```python
from build123d import *

# Parameters (mm, degrees)
F3_W     = 68.58
F3_H     = 68.58
F4_DEPTH = 48.1161598
F7_DEPTH = 203.2


with BuildPart() as f1:
    # F0 (on Front) → F1 (revolve)
    with BuildSketch(Plane.XZ):
        Polygon((228.6, 38.29685), (228.6, 63.5), (197.9639424, 63.5), (191.0935472, 51.6001), (81.237328, 51.6001), (79.8661598, 53.975), (48.1161598, 53.975), (48.1161598, 44.2595), (48.1161598, 38.29685), align=None)
        Polygon((48.1161598, 34.29), (48.1161598, 38.29685), (48.1161598, 44.2595), (0, 44.2595), (0, 34.29), align=None)
    revolve(axis=Axis((114.3, 0, 0), (1, 0, 0)))

    # F3 (on offset) → F4 (cut, through all)
    with BuildSketch(Plane(origin=(0, 0, 0), x_dir=(0, -1, 0), z_dir=(-1, 0, 0))):
        Rectangle(F3_W, F3_H)
    extrude(amount=-F4_DEPTH, mode=Mode.SUBTRACT)

    # F6 (on offset) → F7 (cut, symmetric)
    with BuildSketch(Plane(origin=(48.1161598, 0, 0), x_dir=(0, -1, 0), z_dir=(-1, 0, 0))):
        Polygon((-5.607271922, 5.607271922), (0, 0), (31.9966525594, 31.9966525594), (26.3893806374, 37.6039244814), align=None)
        Polygon((5.607271922, -5.607271922), (0, 0), (-5.607271922, 5.607271922), (-37.6039244814, -26.3893806374), (-26.3893806374, -37.6039244814), align=None)
        Polygon((31.9966525594, 31.9966525594), (0, 0), (5.607271922, -5.607271922), (37.6039244814, 26.3893806374), align=None)
    extrude(amount=F7_DEPTH, both=True, mode=Mode.SUBTRACT)


solid = f1.part
```
Work out the finished part from the listing and answer in its coordinate system (mm). A direction names the side the tool comes from. Give positions to 0.01 mm unless a question says otherwise; leave off trailing zeros. Loops run counter-clockwise (first coordinate to the right, second up) from the corner with the lowest first, then second, coordinate; pieces in that order, holes last. Notation, with made-up numbers: (65.25, 44.25) -> (76.25, 44.25) arc R13 cw to (76.25, 59.25) -> close; hole circle Ø1 at (-26.5, -8). An arc over 180 degrees is marked (long way). Put each result on its own line as item: value. Start each with the question number.
Item 1: Each of these flat-tipped pins is pushed along its axis until it touches: P1, Ø2, axis at y = -37, z = -1, coming from the +X side; P2, Ø3, axis at x = 96.5, y = 4.5, coming from the +Z side; P3, Ø0.7, axis at y = -33, z = 20.5, coming from the -X side. Where does it stop, or does it pass through?
Item 2: The part is cut by section A-A (z = 0). Give the vertices of the cut face in (x, y) (1 decimal), then the cut area to 3 significant figures.
Item 3: Which of the six approach directions +Z, -Z, +X, -X, +Y, -Y give full straight-line access (tool end or side, diameter ignored) to faces 4 (the face through (138.1, 34.814, -23.599)), 5 (the face through (24, -2, -34.29)), 6 (the face through (23.72, 44.24, 1.35)), 7 (the face through (24, 34.29, 2)), 8 (the face through (81.15, 50.52, -11.22))?
Item 4: The mould has two halves that part along Z. Classify faces 1 (the face through (139.62, 27.59, 26.56)), 2 (the face through (135.396, -15.499, 49.217)), 3 (the face through (0, -38, -2)): released by +Z, released by -Z, zero draft, split by the parting line, or undercut.
Item 5: Find the intervals of material crossed by L1, parallel to Y at x = 143.5, z = 2; L2, parallel to Y at x = 68, z = 0.5; L3, parallel to X at y = -25, z = -45, in increasing order. Write a range as [from, to].
Item 6: The part is cut by section D-D (x = 18.5). Give the vertices of the cut face in (y, z).
Item 7: The part is cut by section B-B (x = 166). Give the vertices of the cut face in (y, z).
Answers below:
1. P1: x = 48.12
1. P2: z = 51.51
1. P3: x = 48.12
2. outline: (0, -44.3) -> (48.1, -44.3) -> (48.1, -54) -> (79.9, -54) -> (81.2, -51.6) -> (191.1, -51.6) -> (198, -63.5) -> (228.6, -63.5) -> (228.6, -38.3) -> (48.1, -38.3) -> (48.1, -34.3) -> (0, -34.3) -> close; (0, 34.3) -> (48.1, 34.3) -> (48.1, 38.3) -> (228.6, 38.3) -> (228.6, 63.5) -> (198, 63.5) -> (191.1, 51.6) -> (81.2, 51.6) -> (79.9, 54) -> (48.1, 54) -> (48.1, 44.3) -> (0, 44.3) -> close
2. area: 6,730 mm2
3. face 4: +X, -X
3. face 5: -X, +Y, -Y
3. face 6: -X, +Y
3. face 7: +Z, -Z, -X
3. face 8: none
4. face 1: undercut
4. face 2: split by the parting line
4. face 3: zero draft
5. L1: [-51.56, -38.24], [38.24, 51.56]
5. L2: [-53.97, -38.29], [38.29, 53.97]
5. L3: [48.12, 228.6]
6. outline: (-36.4, 25.18) arc R44.26 ccw to (-34.29, -27.98) -> (-34.29, 23.08) -> close; (-27.98, -34.29) arc R44.26 ccw to (25.18, -36.4) -> (23.08, -34.29) -> close; (-25.18, 36.4) -> (-23.08, 34.29) -> (27.98, 34.29) arc R44.26 ccw to start; (34.29, -23.08) -> (36.4, -25.18) arc R44.26 ccw to (34.29, 27.98) -> close
7. outline: circle Ø103.2 at (0, 0); hole (-37.6, 26.39) -> (-32.1, 20.89) arc R38.3 ccw to (20.89, -32.1) -> (26.39, -37.6) -> (37.6, -26.39) -> (32.1, -20.89) arc R38.3 ccw to (-20.89, 32.1) -> (-26.39, 37.6) -> close
